Input: part model. Units: mm. Frame: model coordinates. A direction names the side the tool comes from. Coordinates: 2 decimals unless noted, no trailing zeros. Loops run counter-clockwise (first coordinate to the right, second up) from the corner with the lowest first, then second, coordinate; pieces in that order, holes last. Notation, with made-up numbers: (53.25, 19.5) -> (91.25, 19.5) arc R29 ccw to (91.25, 42.5) -> close; hole circle Ø7 at (21.25, 38.5). An arc over 180 degrees is marked (long way). Put each result on its own line as item: value. Start each with the question number.
1) Cut plane A-A (x = 69). Return the cut outline in (y, z), plus the area to 3 significant figures.
2) Contact query for flat-ended pins moving along their axis: P1, Ø3, axis at x = 108.5, z = 2.5, coming from the -Y side; P2, Ø2, axis at x = 5, z = 2, coming from the +Y side; P3, Ø2, axis at x = 53.5, z = 2.5, coming from the -Y side. Output: stop coordinate, or through.
3) Cut plane D-D (x = -39.5). Return the cut outline in (y, z).
4) Set-up query: faces 4 (the flat face through (38.456, -40.016, 3.131)), 5 (the flat face through (98, 9, 6.35)). Return all of +Z, -Z, +X, -X, +Y, -Y with unobstructed straight access to the full face (end or side cutting, diameter ignored); none if empty.
5) Pull-direction query (Y, two-part tool) for faces 1 (the cylindrical face through (151.457, 14.248, 3.131)), 2 (the flat face through (98, 9, 0)), 3 (the cylindrical face through (-27.765, -6.784, 3.219)); classes: pulls with the +Y half, pulls with the -Y half, needs draft (parallel to the pull), parting line crosses it, or undercut.
6) Material intervals for L1, parallel to Y at x = 37.5, z = 2.75; L2, parallel to X at y = 32.5, z = 5; L3, parallel to X at y = 4.5, z = 5.5, sorted ascending.
7) Cut plane B-B (y = 60). Return the cut outline in (x, z).
8) Cut plane C-C (z = 4.75). State how many separate pieces and enclosed holes the cut face has, plus the area to 3 significant figures.
from build123d import *

# Parameters (mm, degrees)
SKETCH1_R                 = 107.95
SKETCH1_R_2               = 63.5
BOSS_EXTRUDE1_DEPTH       = 6.35
SKETCH3_R                 = 2.085
CUT_EXTRUDE2_DEPTH        = 229.663768434
CIRPATTERN1_COUNT         = 6
SKETCH4_R                 = 2.085
CUT_EXTRUDE3_DEPTH        = 229.663768434
CIRPATTERN2_COUNT         = 6
SKETCH5_R                 = 2.413
CUT_EXTRUDE4_DEPTH        = 229.663768434
CUT_EXTRUDE7_DEPTH        = 229.663768434
CUT_EXTRUDE7_DEPTH_BACK   = 229.663768434
SKETCH9_R                 = 2.413
CUT_EXTRUDE8_DEPTH        = 229.663768434
CUT_EXTRUDE10_START       = -6.35
CUT_EXTRUDE10_OUTLINE_R   = 3.175
CUT_EXTRUDE10_OUTLINE_R_2 = 2.286
CUT_EXTRUDE10_DEPTH       = 6.35


# Read off the part's stored shape, not the designer's step: Cut-Extrude10
with BuildPart() as part:
    # Sketch1 → Boss-Extrude1 (new body)
    with BuildSketch(Plane.XY):
        with Locations((51.738381467, 55.593319394)):
            Circle(SKETCH1_R)
        with Locations((51.738381467, 55.593319394)):
            Circle(SKETCH1_R_2, mode=Mode.SUBTRACT)
    extrude(amount=BOSS_EXTRUDE1_DEPTH)

    # Sketch3 → Cut-Extrude2 (cut, through all)
    with BuildSketch(Plane.XY.offset(6.35)):
        with Locations((-12.798570104, -22.876686862)):
            Circle(SKETCH3_R)
    cut_extrude2 = extrude(amount=-CUT_EXTRUDE2_DEPTH, mode=Mode.SUBTRACT)

    # CirPattern1: Cut-Extrude2 ×6 about axis
    cirpattern1_axis = Axis((51.738381467, 55.593319394, 0), (0, 0, 1))
    for i in range(1, CIRPATTERN1_COUNT):
        add(cut_extrude2.rotate(cirpattern1_axis, i * 360 / CIRPATTERN1_COUNT), mode=Mode.SUBTRACT)

    # Sketch4 → Cut-Extrude3 (cut, symmetric)
    with BuildSketch(Plane.XY.offset(6.35)):
        with Locations((39.923069121, -10.026449115)):
            Circle(SKETCH4_R)
    cut_extrude3 = extrude(amount=CUT_EXTRUDE3_DEPTH, both=True, mode=Mode.SUBTRACT)

    # CirPattern2: Cut-Extrude3 ×6 about axis
    cirpattern2_axis = Axis((51.738381467, 55.593319394, 0), (0, 0, 1))
    for i in range(1, CIRPATTERN2_COUNT):
        add(cut_extrude3.rotate(cirpattern2_axis, i * 360 / CIRPATTERN2_COUNT), mode=Mode.SUBTRACT)

    # Sketch5 → Cut-Extrude4 (cut, through all)
    with BuildSketch(Plane.XY.offset(6.35)):
        with Locations((-30.066706461, -7.50922857)):
            Circle(SKETCH5_R)
        with Locations((107.725712792, -31.295181319)):
            Circle(SKETCH5_R)
    extrude(amount=-CUT_EXTRUDE4_DEPTH, mode=Mode.SUBTRACT)

    # Sketch8 → Cut-Extrude7 (cut, two sides: drawn at the far end of the back side and taken through both)
    with BuildSketch(Plane.XY.offset(6.35).offset(-CUT_EXTRUDE7_DEPTH_BACK)):
        Polygon((31.650955464, -42.108620026), (32.73112738, -35.85116618), (38.988581226, -36.931338096), (37.90840931, -43.188791942), align=None)
    extrude(amount=CUT_EXTRUDE7_DEPTH + CUT_EXTRUDE7_DEPTH_BACK, mode=Mode.SUBTRACT)

    # Sketch9 → Cut-Extrude8 (cut, through all)
    with BuildSketch(Plane.XY.offset(6.35)):
        with Locations((-3.948592074, 142.429971857)):
            Circle(SKETCH9_R)
        with Locations((133.51515401, 118.700755207)):
            Circle(SKETCH9_R)
    extrude(amount=-CUT_EXTRUDE8_DEPTH, mode=Mode.SUBTRACT)

    # Cut-Extrude10 outline → Cut-Extrude10 (cut)
    with BuildSketch(Plane(origin=(0, 0, 0), x_dir=(-1, 0, 0), z_dir=(0, 0, -1)).offset(CUT_EXTRUDE10_START)):
        with Locations((-148.210776777, 52.562256335)):
            Circle(CUT_EXTRUDE10_OUTLINE_R)
        with Locations((-152.531464441, 77.592071718)):
            Circle(CUT_EXTRUDE10_OUTLINE_R_2)
        with Locations((-150.371120609, 65.077164026)):
            Circle(CUT_EXTRUDE10_OUTLINE_R_2)
    extrude(amount=CUT_EXTRUDE10_DEPTH, mode=Mode.SUBTRACT)


solid = part.part
Results found:
1. outline: (-50.97, 0) -> (-5.52, 0) -> (-5.52, 6.35) -> (-50.97, 6.35) -> close; (116.7, 0) -> (162.15, 0) -> (162.15, 6.35) -> (116.7, 6.35) -> close
1. area: 577 mm2
2. P1: stops at y = -37.14
2. P2: stops at y = 153.37
2. P3: stops at y = -52.35
3. outline: (-2.1, 0) -> (113.29, 0) -> (113.29, 6.35) -> (-2.1, 6.35) -> close
4. face 4: +Z, -Z
4. face 5: +Z, +X, -X, +Y, -Y
5. face 1: parting line crosses it
5. face 2: needs draft
5. face 3: undercut
6. L1: y = -51.41 to -43.12, -36.67 to -6.29, 117.48 to 162.6
6. L2: x = -53.71 to -13.02, -8.98 to -7.41, 110.89 to 157.19
6. L3: x = -43.35 to 14.03, 89.44 to 146.83
7. outline: (-56.12, 0) -> (-11.61, 0) -> (-11.61, 6.35) -> (-56.12, 6.35) -> close; (115.09, 0) -> (159.6, 0) -> (159.6, 6.35) -> (115.09, 6.35) -> close
8. separate pieces: 1
8. enclosed holes: 21
8. area: 23,600 mm2
